```python
from build123d import *

# Parameters (mm, degrees)
F0_R      = 285.75
F1_DEPTH  = 1.27
F2_R      = 285.75
F2_R_2    = 285.115
F3_DEPTH  = 869.95
F4_R      = 234.95
F4_R_2    = 234.315
F5_DEPTH  = 869.95
F6_R      = 208.915
F6_R_2    = 208.28
F7_DEPTH  = 869.95
F9_DEPTH  = 285.751
F11_DEPTH = 304.8


with BuildPart() as f1:
    # F0 (on Top) → F1 (new body)
    with BuildSketch(Plane.XY):
        Circle(F0_R)
    extrude(amount=-F1_DEPTH)

    # F2 (on face) → F3 (join)
    with BuildSketch(Plane.XY):
        Circle(F2_R)
        Circle(F2_R_2, mode=Mode.SUBTRACT)
    extrude(amount=F3_DEPTH)

    # F4 (on face) → F5 (join)
    with BuildSketch(Plane.XY):
        Circle(F4_R)
        Circle(F4_R_2, mode=Mode.SUBTRACT)
    extrude(amount=F5_DEPTH)

    # F6 (on face) → F7 (join)
    with BuildSketch(Plane.XY):
        Circle(F6_R)
        Circle(F6_R_2, mode=Mode.SUBTRACT)
    extrude(amount=F7_DEPTH)

    # F8 (on Front) → F9 (cut, through all)
    with BuildSketch(Plane.XZ):
        with BuildLine():
            ThreePointArc((0, 0.635), (24.695704, 10.864296), (34.925, 35.56))
            ThreePointArc((34.925, 35.56), (-24.695704, 60.255704), (0, 0.635))
        make_face()
    extrude(amount=F9_DEPTH, mode=Mode.SUBTRACT)

    # F10 (on Right) → F11 (cut)
    with BuildSketch(Plane.YZ):
        Polygon((-152.4, 76.2), (0, 76.2), (152.4, 76.2), (152.4, 228.6), (-152.4, 228.6), align=None)
    extrude(amount=F11_DEPTH, mode=Mode.SUBTRACT)


solid = f1.part
```
CAD build for the part. Positions are in the model's coordinates, mm. Coordinates: 2 decimals unless noted, no trailing zeros. Order: outer loops, then holes, each group sorted by start corner. A loop starts at its lowest first (then second) coordinate and runs counter-clockwise, first axis right, second up. Notation, with made-up numbers: (54, 11.25) - (61, 11.25) arc R29 ccw to (61, 42.25) - close; hole circle Ø5 at (-37, 7.5). An arc over 180 degrees is marked (long way). Use a Markdown table: item, result. Add a question column.
(1) Pull direction X, two halves, no side cores. Call faces 1 (the face through (-234.723, 10.33, 428.885)), 2 (the face through (-4, 4, -1.27)): +X half, -X half, draft (parallel to the pull), parting line (faces both ways), or undercut.
(2) Flat gauge pins, fed straight in: pin 1 (0.7 mm diameter, centred on x = 178.5, z = 163, fed in from -Y); pin 2 (0.9 mm diameter, centred on x = 178.5, z = 154, fed in from +Y); pin 3 (0.6 mm diameter, centred on x = 241.5, z = 161.5, fed in from -Y). Where does each tip first touch, or does it go through?
(3) Saw through at D-D (x = -80). Give the cut face in (y, z).
(4) Saw through at A-A (z = 685.5). Give the cut face in (x, y) (3 decimals), then the cut area to 3 significant figures.
(5) Drill centre lines: line 1 along Y through (x, z) = (0, 461) (3 decimals); line 2 along Y through (x, z) = (146.5, 711.5); line 3 along X through (y, z) = (193, 479.5). Where is each one in solid material? Low to high. Write a range as [from, to].
(6) Saw through at B-B (z = 182). Give the cut face in (x, y) (3 decimals).
Solved:
| question | item | result |
|---|---|---|
| 1 | face 1 | undercut |
| 1 | face 2 | draft |
| 2 | pin 1 | stops at y = -223.42 |
| 2 | pin 2 | stops at y = 223.5 |
| 2 | pin 3 | stops at y = -153.22 |
| 3 | outline | (-274.32, -1.27) - (274.32, -1.27) - (274.32, 869.95) - (273.66, 869.95) - (273.66, 0) - (220.91, 0) - (220.91, 869.95) - (220.24, 869.95) - (220.24, 0) - (192.99, 0) - (192.99, 869.95) - (192.3, 869.95) - (192.3, 0) - (-192.3, 0) - (-192.3, 869.95) - (-192.99, 869.95) - (-192.99, 0) - (-220.24, 0) - (-220.24, 869.95) - (-220.91, 869.95) - (-220.91, 0) - (-273.66, 0) - (-273.66, 869.95) - (-274.32, 869.95) - close |
| 4 | outline | circle Ø571.5 at (0, 0); circle Ø469.9 at (0, 0); circle Ø417.83 at (0, 0); hole circle Ø570.23 at (0, 0); hole circle Ø468.63 at (0, 0); hole circle Ø416.56 at (0, 0) |
| 4 | area | 2,910 mm² |
| 5 | line 1 | y = [-285.75, -285.115], [-234.95, -234.315], [-208.915, -208.28], [208.28, 208.915], [234.315, 234.95], [285.115, 285.75] |
| 5 | line 2 | y = [-245.34, -244.6], [-183.68, -182.87], [-148.94, -148.05], [148.05, 148.94], [182.87, 183.68], [244.6, 245.34] |
| 5 | line 3 | x = [-210.72, -209.86], [-133.99, -132.87], [-79.98, -78.3], [78.3, 79.98], [132.87, 133.99], [209.86, 210.72] |
| 6 | outline | (141.968, -152.4) arc R208.28 cw (long way) to (141.968, 152.4) - (142.898, 152.4) arc R208.915 ccw (long way) to (142.898, -152.4) - close; (177.982, -152.4) arc R234.315 cw (long way) to (177.982, 152.4) - (178.818, 152.4) arc R234.95 ccw (long way) to (178.818, -152.4) - close; (240.966, -152.4) arc R285.115 cw (long way) to (240.966, 152.4) - (241.717, 152.4) arc R285.75 ccw (long way) to (241.717, -152.4) - close |
